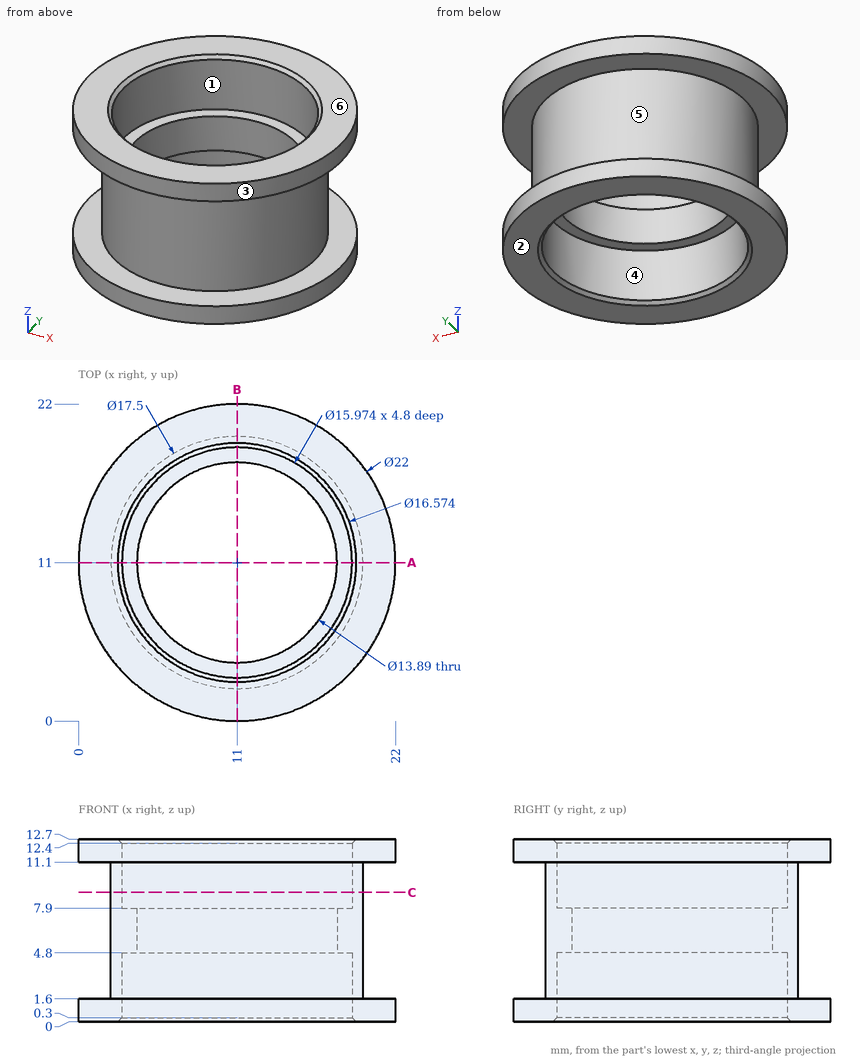
Answer from the drawing. Dimensions are ordinates in mm from the lowest x, y and z of the part. A direction names the side the tool comes from. Coordinates: 2 decimals unless noted, no trailing zeros. Write each loop counter-clockwise with the first axis right and the second up, starting at its lowest first coordinate (ties: lowest second). Pieces come first, ordered by that corner, then holes. Notation, with made-up numbers: M -25,-36 L -3,-36 A28 ccw -3,0 Z; hole C 26.5,-23 d8. An arc over 180 degrees is marked long. Write item = value, one per line.
1. For the marked faces 4, 5 and 6, determine the directions among +Z, -Z, +X, -X, +Y, -Y from which every point of the face is accessible in a straight line to the end or side of a thin tool.
Solution:
face_4 = -Z
face_5 = none
face_6 = +Z, +X, -X, +Y, -Y
2. The part is cut by section C-C (z = 9). Determine the outline of the cut face in (x, y).
Solution:
outline = C 11,11 d17.5; hole C 11,11 d15.97
3. The part is cut by section A-A (y = 11). Determine the outline of the cut face in (x, z) (3 decimals).
Solution:
outline = M 0,0 L 2.713,0 L 3.013,0.3 L 3.013,4.8 L 4.055,4.8 L 4.055,7.9 L 3.013,7.9 L 3.013,12.4 L 2.713,12.7 L 0,12.7 L 0,11.1 L 2.25,11.1 L 2.25,1.6 L 0,1.6 Z; M 17.945,4.8 L 18.987,4.8 L 18.987,0.3 L 19.287,0 L 22,0 L 22,1.6 L 19.75,1.6 L 19.75,11.1 L 22,11.1 L 22,12.7 L 19.287,12.7 L 18.987,12.4 L 18.987,7.9 L 17.945,7.9 Z
4. Straight lines are drawn through the part: line 1 (X direction, y = 11, z = 9.5); line 2 (Z direction, x = 2.75, y = 16.5); line 3 (X direction, y = 11, z = 6.3) (3 decimals). For each, find the intervals that lie inside material, in ascending order. Write a range as from..to.
Solution:
line_1 = 2.25..3.01, 18.99..19.75
line_2 = 0..1.6, 11.1..12.7
line_3 = 2.25..4.055, 17.945..19.75
5. Determine the mould class of the marked faces 1, 2 and 3 for opening direction X: released by +X, released by -X, zero draft, split by the parting line, or undercut.
Solution:
face_1 = undercut
face_2 = zero draft
face_3 = split by the parting line
6. Flat-ended cylindrical pins translate along their axes: pin 1 (1 mm diameter, centred on y = 15.5, z = 1.5, fed in from -X); pin 2 (1 mm diameter, centred on y = 6.5, z = 7.5, fed in from -X); pin 3 (4 mm diameter, centred on x = 18.5, z = 2, fed in from +Y). Find the tip coordinate at first contact, or state that the pin passes through.
Solution:
pin_1 = 0.75
pin_2 = 3.22
pin_3 = 20.5
